For this review, take the finished solid that the model builds, in its own axes (mm). A direction names the side the tool comes from. Coordinates: 2 decimals unless noted, no trailing zeros. Loops run counter-clockwise (first coordinate to the right, second up) from the corner with the lowest first, then second, coordinate; pieces in that order, holes last.
```python
from build123d import *

# Parameters (mm, degrees)
F0_W     = 1880
F0_H     = 910
F1_DEPTH = 500
F2_W     = 350
F2_H     = 700
F3_DEPTH = 100
F4_R     = 25
F5_R     = 50


with BuildPart() as f1:
    # F0 (on Top) → F1 (new body)
    with BuildSketch(Plane.XY):
        with Locations((940, 455)):
            Rectangle(F0_W, F0_H)
    extrude(amount=F1_DEPTH)

    # F2 (on face) → F3 (join)
    with BuildSketch(Plane.XY.offset(500)):
        with Locations((225, 455)):
            Rectangle(F2_W, F2_H)
    extrude(amount=F3_DEPTH)

    # F4
    f4_edges = [f1.edges().sort_by_distance(p)[0] for p in [
        (50, 455, 600),
        (225, 105, 600),
        (400, 455, 600),
        (225, 805, 600),
    ]]
    fillet(f4_edges, radius=F4_R)

    # F5
    f5_edges = [f1.edges().sort_by_distance(p)[0] for p in [
        (940, 910, 500),
        (1880, 455, 500),
        (940, 0, 500),
    ]]
    fillet(f5_edges, radius=F5_R)


solid = f1.part
```
Q1. For pin 1 Ø8 at (x, z) = (561, 487.5) entering from +Y; pin 2 Ø12 at (x, y) = (1653, 318) entering from +Z; pin 3 Ø22.5 at (x, z) = (163.5, 522) entering from -Y, all flat-tipped, find the tip position at first contact; note any pin that passes through.
Q2. Consider section B-B (x = 126.5). State the section outline as (y, z) points, then the cut area to 3 significant figures.
Q3. Machinability: for faces 1 (the face through (927, 0, 222)), 2 (the face through (223, 805, 537)), 3 (the face through (223, 105, 537)), 4 (the face through (50, 450, 537)), 5 (the face through (400, 450, 537)), which of the approach directions +Z, -Z, +X, -X, +Y, -Y give a long, thin tool a straight path to every point of the face, cutting with its end or side? Answer none if there is none.
Q4. Consider section C-C (x = 1220). State the section outline as (y, z) points, then the cut area to 3 significant figures.
Q5. Wall thickness on probe 1 along Z at (x, y) = (459.5, 861); probe 2 along X at (y, z) = (581.5, 525); probe 3 along Y at (x, z) = (1562.5, 461) (3 decimals): over which ranges is each line inside the solid? List them lowest first.
Q6. Consider section A-A (y = 647.5). State the section outline as (x, z) points, then the cut area to 3 significant figures.
Model answer:
1. pin 1: stops at y = 897.12
1. pin 2: stops at z = 500
1. pin 3: stops at y = 105
2. outline: (0, 0) - (910, 0) - (910, 450) arc R50 ccw to (860, 500) - (805, 500) - (805, 575) arc R25 ccw to (780, 600) - (130, 600) arc R25 ccw to (105, 575) - (105, 500) - (50, 500) arc R50 ccw to (0, 450) - close
2. area: 524,000 mm2
3. face 1: +Z, -Z, +X, -X, -Y
3. face 2: +Z, +X, -X, +Y
3. face 3: +Z, +X, -X, -Y
3. face 4: +Z, -X, +Y, -Y
3. face 5: +Z, +X, +Y, -Y
4. outline: (0, 0) - (910, 0) - (910, 450) arc R50 ccw to (860, 500) - (50, 500) arc R50 ccw to (0, 450) - close
4. area: 454,000 mm2
5. probe 1: z = 0 to 499.99
5. probe 2: x = 50 to 400
5. probe 3: y = 1.225 to 908.775
6. outline: (0, 0) - (1880, 0) - (1880, 450) arc R50 ccw to (1830, 500) - (400, 500) - (400, 575) arc R25 ccw to (375, 600) - (75, 600) arc R25 ccw to (50, 575) - (50, 500) - (0, 500) - close
6. area: 974,000 mm2
